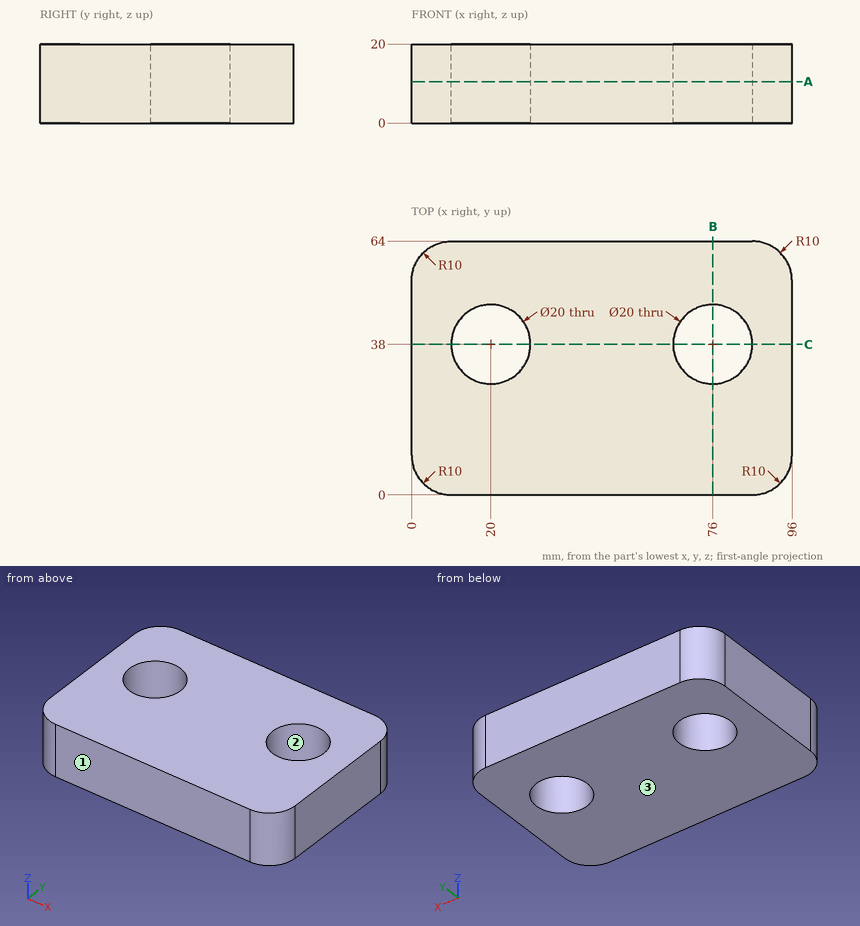
Design review of the part shown in the three views and the two pictorial views. Dimensions are in mm from the part's minimum x, y and z. Round coordinates to 2 decimals unless told otherwise and drop trailing zeros. Loops run counter-clockwise (first coordinate to the right, second up) from the corner with the lowest first, then second, coordinate; pieces in that order, holes last.
(1) Wall thickness on line 1 along Y through (x, z) = (20, 9.5); line 2 along X through (y, z) = (47, 10.75); line 3 along Y through (x, z) = (84.5, 14.5): over which ranges is each line inside the solid? List them lowest first.
Returned:
line 1: y = 0 to 28, 48 to 64
line 2: x = 0 to 15.64, 24.36 to 71.64, 80.36 to 96
line 3: y = 0 to 32.73, 43.27 to 64
(2) We need section A-A (z = 10.5). Give the boundary of the cut face in (x, y).
Returned:
outline: (0, 10) arc R10 ccw to (10, 0) - (86, 0) arc R10 ccw to (96, 10) - (96, 54) arc R10 ccw to (86, 64) - (10, 64) arc R10 ccw to (0, 54) - close; hole circle Ø20 at (20, 38); hole circle Ø20 at (76, 38)
(3) Mouldability with a two-part tool opening along Y and no side actions: class the marked faces 1, 2 and 3 as released by +Y, released by -Y, zero draft, split by the parting line, or undercut.
Returned:
face 1: released by -Y
face 2: undercut
face 3: zero draft
(4) We need section B-B (x = 76). Give the boundary of the cut face in (y, z), plus the area to 3 significant figures.
Returned:
outline: (0, 0) - (28, 0) - (28, 20) - (0, 20) - close; (48, 0) - (64, 0) - (64, 20) - (48, 20) - close
area: 880 mm2
(5) We need section C-C (y = 38). Give the boundary of the cut face in (x, z), plus the area to 3 significant figures.
Returned:
outline: (0, 0) - (10, 0) - (10, 20) - (0, 20) - close; (30, 0) - (66, 0) - (66, 20) - (30, 20) - close; (86, 0) - (96, 0) - (96, 20) - (86, 20) - close
area: 1,120 mm2
